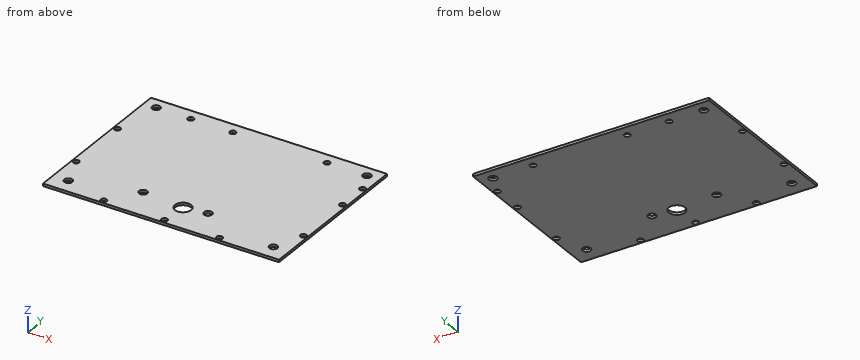
```python
from build123d import *

# Parameters (mm, degrees)
SKETCH1_W           = 148.59
SKETCH1_H           = 106.68
BOSS_EXTRUDE1_DEPTH = 1.5875
SKETCH2_R           = 2.54
CUT_EXTRUDE1_DEPTH  = 2.5875
CUT_EXTRUDE2_REACH  = 3.587
SKETCH3_R           = 5.08
CUT_EXTRUDE3_REACH  = 3.587
SKETCH4_R           = 1.905
CUT_EXTRUDE4_REACH  = 3.587
SKETCH5_R           = 2.54


with BuildPart() as part:
    # Sketch1 → Boss-Extrude1 (new body)
    with BuildSketch(Plane.XY):
        Rectangle(SKETCH1_W, SKETCH1_H)
    extrude(amount=BOSS_EXTRUDE1_DEPTH)

    # Sketch2 → Cut-Extrude1 (cut, through all)
    with BuildSketch(Plane.XY.offset(1.5875)):
        with Locations((-64.5325, -43.5775)):
            Circle(SKETCH2_R)
        with Locations((64.5325, -43.5775)):
            Circle(SKETCH2_R)
        with Locations((-66.3575, 46.0375)):
            Circle(SKETCH2_R)
        with Locations((66.3575, 46.0375)):
            Circle(SKETCH2_R)
    extrude(amount=-CUT_EXTRUDE1_DEPTH, mode=Mode.SUBTRACT)

    # Sketch3 → Cut-Extrude2 (cut, up to next)
    with BuildSketch(Plane.XY.offset(1.5875), mode=Mode.PRIVATE) as cut_extrude2_sk1:
        with Locations((1.905, -34.544)):
            Circle(SKETCH3_R)
    cut_extrude2_tool1 = extrude(cut_extrude2_sk1.sketch, amount=-CUT_EXTRUDE2_REACH, mode=Mode.PRIVATE) & part.part
    add(cut_extrude2_tool1.solids().sort_by_distance((1.905, -34.544, 1.5875))[0], mode=Mode.SUBTRACT)

    # Sketch4 → Cut-Extrude3 (cut, up to next)
    with BuildSketch(Plane.XY.offset(1.5875), mode=Mode.PRIVATE) as cut_extrude3_sk1:
        with Locations((-44.578582342, 46.016934616)):
            Circle(SKETCH4_R)
    cut_extrude3_tool1 = extrude(cut_extrude3_sk1.sketch, amount=-CUT_EXTRUDE3_REACH, mode=Mode.PRIVATE) & part.part
    add(cut_extrude3_tool1.solids().sort_by_distance((-44.578582, 46.016935, 1.5875))[0], mode=Mode.SUBTRACT)
    # Sketch4 → Cut-Extrude3 (cut, up to next)
    with BuildSketch(Plane.XY.offset(1.5875), mode=Mode.PRIVATE) as cut_extrude3_sk2:
        with Locations((-18.096274256, 46.016934616)):
            Circle(SKETCH4_R)
    cut_extrude3_tool2 = extrude(cut_extrude3_sk2.sketch, amount=-CUT_EXTRUDE3_REACH, mode=Mode.PRIVATE) & part.part
    add(cut_extrude3_tool2.solids().sort_by_distance((-18.096274, 46.016935, 1.5875))[0], mode=Mode.SUBTRACT)
    # Sketch4 → Cut-Extrude3 (cut, up to next)
    with BuildSketch(Plane.XY.offset(1.5875), mode=Mode.PRIVATE) as cut_extrude3_sk3:
        with Locations((41.222617745, 46.016934616)):
            Circle(SKETCH4_R)
    cut_extrude3_tool3 = extrude(cut_extrude3_sk3.sketch, amount=-CUT_EXTRUDE3_REACH, mode=Mode.PRIVATE) & part.part
    add(cut_extrude3_tool3.solids().sort_by_distance((41.222618, 46.016935, 1.5875))[0], mode=Mode.SUBTRACT)
    # Sketch4 → Cut-Extrude3 (cut, up to next)
    with BuildSketch(Plane.XY.offset(1.5875), mode=Mode.PRIVATE) as cut_extrude3_sk4:
        with Locations((71.795, 33.199680415)):
            Circle(SKETCH4_R)
    cut_extrude3_tool4 = extrude(cut_extrude3_sk4.sketch, amount=-CUT_EXTRUDE3_REACH, mode=Mode.PRIVATE) & part.part
    add(cut_extrude3_tool4.solids().sort_by_distance((71.795, 33.19968, 1.5875))[0], mode=Mode.SUBTRACT)
    # Sketch4 → Cut-Extrude3 (cut, up to next)
    with BuildSketch(Plane.XY.offset(1.5875), mode=Mode.PRIVATE) as cut_extrude3_sk5:
        with Locations((71.795, 13.37524336)):
            Circle(SKETCH4_R)
    cut_extrude3_tool5 = extrude(cut_extrude3_sk5.sketch, amount=-CUT_EXTRUDE3_REACH, mode=Mode.PRIVATE) & part.part
    add(cut_extrude3_tool5.solids().sort_by_distance((71.795, 13.375243, 1.5875))[0], mode=Mode.SUBTRACT)
    # Sketch4 → Cut-Extrude3 (cut, up to next)
    with BuildSketch(Plane.XY.offset(1.5875), mode=Mode.PRIVATE) as cut_extrude3_sk6:
        with Locations((71.795, -25.245906802)):
            Circle(SKETCH4_R)
    cut_extrude3_tool6 = extrude(cut_extrude3_sk6.sketch, amount=-CUT_EXTRUDE3_REACH, mode=Mode.PRIVATE) & part.part
    add(cut_extrude3_tool6.solids().sort_by_distance((71.795, -25.245907, 1.5875))[0], mode=Mode.SUBTRACT)
    # Sketch4 → Cut-Extrude3 (cut, up to next)
    with BuildSketch(Plane.XY.offset(1.5875), mode=Mode.PRIVATE) as cut_extrude3_sk7:
        with Locations((35.197381877, -50.84)):
            Circle(SKETCH4_R)
    cut_extrude3_tool7 = extrude(cut_extrude3_sk7.sketch, amount=-CUT_EXTRUDE3_REACH, mode=Mode.PRIVATE) & part.part
    add(cut_extrude3_tool7.solids().sort_by_distance((35.197382, -50.84, 1.5875))[0], mode=Mode.SUBTRACT)
    # Sketch4 → Cut-Extrude3 (cut, up to next)
    with BuildSketch(Plane.XY.offset(1.5875), mode=Mode.PRIVATE) as cut_extrude3_sk8:
        with Locations((0.59225822, -50.84)):
            Circle(SKETCH4_R)
    cut_extrude3_tool8 = extrude(cut_extrude3_sk8.sketch, amount=-CUT_EXTRUDE3_REACH, mode=Mode.PRIVATE) & part.part
    add(cut_extrude3_tool8.solids().sort_by_distance((0.592258, -50.84, 1.5875))[0], mode=Mode.SUBTRACT)
    # Sketch4 → Cut-Extrude3 (cut, up to next)
    with BuildSketch(Plane.XY.offset(1.5875), mode=Mode.PRIVATE) as cut_extrude3_sk9:
        with Locations((-37.65546217, -50.84)):
            Circle(SKETCH4_R)
    cut_extrude3_tool9 = extrude(cut_extrude3_sk9.sketch, amount=-CUT_EXTRUDE3_REACH, mode=Mode.PRIVATE) & part.part
    add(cut_extrude3_tool9.solids().sort_by_distance((-37.655462, -50.84, 1.5875))[0], mode=Mode.SUBTRACT)
    # Sketch4 → Cut-Extrude3 (cut, up to next)
    with BuildSketch(Plane.XY.offset(1.5875), mode=Mode.PRIVATE) as cut_extrude3_sk10:
        with Locations((-71.823750006, -24.517485795)):
            Circle(SKETCH4_R)
    cut_extrude3_tool10 = extrude(cut_extrude3_sk10.sketch, amount=-CUT_EXTRUDE3_REACH, mode=Mode.PRIVATE) & part.part
    add(cut_extrude3_tool10.solids().sort_by_distance((-71.82375, -24.517486, 1.5875))[0], mode=Mode.SUBTRACT)
    # Sketch4 → Cut-Extrude3 (cut, up to next)
    with BuildSketch(Plane.XY.offset(1.5875), mode=Mode.PRIVATE) as cut_extrude3_sk11:
        with Locations((-71.823750006, 16.385688775)):
            Circle(SKETCH4_R)
    cut_extrude3_tool11 = extrude(cut_extrude3_sk11.sketch, amount=-CUT_EXTRUDE3_REACH, mode=Mode.PRIVATE) & part.part
    add(cut_extrude3_tool11.solids().sort_by_distance((-71.82375, 16.385689, 1.5875))[0], mode=Mode.SUBTRACT)

    # Sketch5 → Cut-Extrude4 (cut, up to next)
    with BuildSketch(Plane.XY.offset(1.5875), mode=Mode.PRIVATE) as cut_extrude4_sk1:
        with Locations((-24.584832927, -32.40931441)):
            Circle(SKETCH5_R)
    cut_extrude4_tool1 = extrude(cut_extrude4_sk1.sketch, amount=-CUT_EXTRUDE4_REACH, mode=Mode.PRIVATE) & part.part
    add(cut_extrude4_tool1.solids().sort_by_distance((-24.584833, -32.409314, 1.5875))[0], mode=Mode.SUBTRACT)
    # Sketch5 → Cut-Extrude4 (cut, up to next)
    with BuildSketch(Plane.XY.offset(1.5875), mode=Mode.PRIVATE) as cut_extrude4_sk2:
        with Locations((16.415053576, -32.617647841)):
            Circle(SKETCH5_R)
    cut_extrude4_tool2 = extrude(cut_extrude4_sk2.sketch, amount=-CUT_EXTRUDE4_REACH, mode=Mode.PRIVATE) & part.part
    add(cut_extrude4_tool2.solids().sort_by_distance((16.415054, -32.617648, 1.5875))[0], mode=Mode.SUBTRACT)


solid = part.part
```
The model under review builds one solid part; all positions refer to its coordinate system, in mm. Round coordinates to 2 decimals unless told otherwise and drop trailing zeros. Loops run counter-clockwise (first coordinate to the right, second up) from the corner with the lowest first, then second, coordinate; pieces in that order, holes last.
Item 1: Take a section at B-B (z = 0.6). Give the number of separate pieces and of enclosed holes in the cut face, then the cut area to 3 significant figures.
Determined:
separate pieces: 1
enclosed holes: 18
area: 15,500 mm2
Item 2: Clearance check with a flat-ended pin moving along its axis: pin 1 Ø3.5 at (x, y) = (0.59, -50.84) entering from +Z. State where the tip first meets the part, or that it passes through.
Determined:
pin 1: passes through
Item 3: For line 1 (X direction, y = -43.5, z = 0.55) (3 decimals); line 2 (X direction, y = 13, z = 0.95) (3 decimals); line 3 (Y direction, x = 66, z = 1.05), list the stretches that pass through material, from the lowest coordinate up.
Determined:
line 1: x = -74.295 to -67.071, -61.994 to 61.994, 67.071 to 74.295
line 2: x = -74.295 to 69.927, 73.663 to 74.295
line 3: y = -53.34 to -45.65, -41.5 to 43.52, 48.55 to 53.34
Item 4: Take a section at A-A (y = -50.84). Write out the cut boundary in (x, z) (1 decimal), then the cut area to 3 significant figures.
Determined:
outline: (-74.3, 0) - (-39.6, 0) - (-39.6, 1.6) - (-74.3, 1.6) - close; (-35.8, 0) - (-1.3, 0) - (-1.3, 1.6) - (-35.8, 1.6) - close; (2.5, 0) - (33.3, 0) - (33.3, 1.6) - (2.5, 1.6) - close; (37.1, 0) - (74.3, 0) - (74.3, 1.6) - (37.1, 1.6) - close
area: 218 mm2
